Read the model definition and answer for the solid it produces. Units are mm, in the model's axes. A direction names the side the tool comes from. Coordinates: 2 decimals unless noted, no trailing zeros.
from build123d import *

# Parameters (mm, degrees)
F1_DEPTH = 5.08
F2_SIZE  = 5.07999
F3_R     = 2.54


# Not quite as in the source:
# - a fillet or chamfer is up to 0.001 mm smaller than in the source, because OpenCascade refuses the exact size


with BuildPart() as f1:
    # F0 (on Top) → F1 (new body)
    with BuildSketch(Plane.XY):
        Polygon((-50.5690909922, 21.4745439589), (-59.1589100659, 21.4745439589), (-59.2091714259, 13.8599455538), (-59.4360008836, -20.5047279596), (-50.5690909922, -20.5047279596), (-50.5690909922, 14.3012451008), align=None)
        with BuildLine():
            Line((-59.2091714259, 13.8599455538), (-59.1589100659, 21.4745439589))
            Line((-59.1589100659, 21.4745439589), (-64.0080049634, 21.4745439589))
            add(Edge.make_bspline(
                [(-64.0080049634, 21.4745439589), (-63.0207799447, 20.8576332232), (-60.7789769957, 19.4567445904), (-59.7724519982, 15.8681994581), (-59.2091714259, 13.8599455538)],
                knots=[0, 0, 0, 0, 0.4403710055, 1, 1, 1, 1], degree=3))
        make_face()
        Polygon((-59.1589100659, 47.79817909), (-59.1589100659, 21.4745439589), (-50.5690909922, 21.4745439589), (-50.5690909922, 64.423635602), align=None)
        with BuildLine():
            Line((-45.6602349877, 21.4745439589), (-50.5690909922, 21.4745439589))
            Line((-50.5690909922, 21.4745439589), (-50.5690909922, 14.3012451008))
            add(Edge.make_bspline(
                [(-45.6602349877, 21.4745439589), (-46.6065278441, 20.9184128466), (-48.770914008, 19.6464149903), (-49.9215342609, 16.2261394646), (-50.5690909922, 14.3012451008)],
                knots=[0, 0, 0, 0, 0.4372107307, 1, 1, 1, 1], degree=3))
        make_face()
    extrude(amount=F1_DEPTH)

    # F2 (size 5.08 in the source; OpenCascade refuses exactly that, so slightly less here)
    f2_edges = [f1.edges().sort_by_distance(p)[0] for p in [
        (-59.15891, 34.636362, 5.08),
        (-54.864001, 56.110907, 5.08),
    ]]
    chamfer(f2_edges, length=F2_SIZE)

    # F3
    f3_edges = [f1.edges().sort_by_distance(p)[0] for p in [
        (-59.322586, -3.322391, 5.08),
        (-50.569091, -3.101741, 5.08),
        (-60.725717, 18.263642, 5.08),
        (-48.908594, 18.46974, 5.08),
    ]]
    fillet(f3_edges, radius=F3_R)


solid = f1.part
Q1. Which of the six approach directions +Z, -Z, +X, -X, +Y, -Y give full straight-line access (tool end or side, diameter ignored) to faces 1 (the cylindrical face through (-51.293, -2.647, 4.316)), 2 (the flat face through (-50.569, 38, 3)), 3 (the flat face through (-56.58, 34.82, 2.58))?
Q2. Determine the mould class of faces 4 (the flat face through (-55, 23, 0)), 5 (the flat face through (-48, 21.475, 3)), 6 (the cylindrical face through (-58.599, -3.391, 4.316)), 7 (the flat face through (-55, -20.505, 3)) for opening direction Y: +Y half, -Y half, draft (parallel to the pull), parting line (faces both ways), or undercut.
Q3. Each of these flat-tipped pins is pushed along its axis until it touches: P1, Ø2, axis at x = -49, y = 49, coming from the +Z side; P2, Ø0.8, axis at y = -1.5, z = 1, coming from the +X side; P3, Ø2, axis at x = -62, y = 19, coming from the +Z side. Where does it stop, or does it pass through?
Q4. Straight lines are drawn through the part: L1, parallel to Y at x = -58.5, z = 2.4; L2, parallel to X at y = 30.5, z = 2.5; L3, parallel to X at y = 27.5, z = 1.4. For each, find the intervals that lie inside material, in ascending order.
Computed values:
1. face 1: +Z, +X, -Y
1. face 2: +Z, -Z, +X, +Y
1. face 3: +Z, -X, +Y
2. face 4: draft
2. face 5: +Y half
2. face 6: undercut
2. face 7: -Y half
3. P1: passes through
3. P2: stops at x = -50.57
3. P3: stops at z = 3.76
4. L1: y = -20.5 to 21.47
4. L2: x = -56.66 to -50.57
4. L3: x = -57.76 to -50.57
